```python
from build123d import *

# Parameters (mm, degrees)
SKETCH1_W           = 125
SKETCH1_H           = 6
BOSS_EXTRUDE1_DEPTH = 4
SKETCH2_R           = 1.15
CUT_EXTRUDE1_DEPTH  = 4
SKETCH4_W           = 6
SKETCH4_H           = 6
BOSS_EXTRUDE2_DEPTH = 10
SKETCH5_R           = 1.25
CUT_EXTRUDE2_DEPTH  = 10
SKETCH6_W           = 125
SKETCH6_H           = 6
CUT_EXTRUDE3_DEPTH  = 2
SKETCH7_R           = 1.5
CUT_EXTRUDE5_DEPTH  = 2
SKETCH8_R           = 1.5
CUT_EXTRUDE6_DEPTH  = 10
SKETCH9_R           = 1.5
CUT_EXTRUDE7_DEPTH  = 10
SKETCH10_W          = 6
SKETCH10_H          = 2
CUT_EXTRUDE8_DEPTH  = 20
SKETCH11_R          = 1.5
BOSS_EXTRUDE3_DEPTH = 2
SKETCH12_R          = 1.5
CUT_EXTRUDE9_DEPTH  = 2


with BuildPart() as part:
    # Sketch1 → Boss-Extrude1 (new body)
    with BuildSketch(Plane(origin=(0, 0, 0), x_dir=(1, 0, 0), z_dir=(0, 1, 0))):
        Rectangle(SKETCH1_W, SKETCH1_H)
    extrude(amount=BOSS_EXTRUDE1_DEPTH)

    # Sketch2 → Cut-Extrude1 (cut)
    with BuildSketch(Plane.XZ):
        with Locations(Location((0, 0, 0), (0, 0, 270))):
            Circle(SKETCH2_R)
    extrude(amount=-CUT_EXTRUDE1_DEPTH, mode=Mode.SUBTRACT)

    # Sketch4 → Boss-Extrude2 (add)
    with BuildSketch(Plane(origin=(62.5, 0, 0), x_dir=(0, 0, -1), z_dir=(1, 0, 0))):
        with Locations((0, 3)):
            Rectangle(SKETCH4_W, SKETCH4_H)
    extrude(amount=BOSS_EXTRUDE2_DEPTH)

    # Sketch5 → Cut-Extrude2 (cut)
    with BuildSketch(Plane(origin=(72.5, 0, 0), x_dir=(0, 0, -1), z_dir=(1, 0, 0))):
        with Locations((0, 3)):
            Circle(SKETCH5_R)
    extrude(amount=-CUT_EXTRUDE2_DEPTH, mode=Mode.SUBTRACT)

    # Sketch6 → Cut-Extrude3 (cut)
    with BuildSketch(Plane(origin=(0, 4, 0), x_dir=(1, 0, 0), z_dir=(0, 1, 0))):
        Rectangle(SKETCH6_W, SKETCH6_H)
    extrude(amount=-CUT_EXTRUDE3_DEPTH, mode=Mode.SUBTRACT)

    # Sketch7 → Cut-Extrude5 (cut)
    with BuildSketch(Plane(origin=(0, 2, 0), x_dir=(1, 0, 0), z_dir=(0, 1, 0))):
        with Locations(Location((0, 0, 0), (0, 0, 270))):
            Circle(SKETCH7_R)
    extrude(amount=-CUT_EXTRUDE5_DEPTH, mode=Mode.SUBTRACT)

    # Sketch8 → Cut-Extrude6 (cut)
    with BuildSketch(Plane(origin=(72.5, 0, 0), x_dir=(0, 0, -1), z_dir=(1, 0, 0))):
        with Locations((0, 3)):
            Circle(SKETCH8_R)
    extrude(amount=-CUT_EXTRUDE6_DEPTH, mode=Mode.SUBTRACT)

    # Sketch9 → Cut-Extrude7 (cut)
    with BuildSketch(Plane(origin=(0, 2, 0), x_dir=(1, 0, 0), z_dir=(0, 1, 0))):
        with Locations(Location((-57.5, 0, 0), (0, 0, 270))):
            Circle(SKETCH9_R)
    extrude(amount=-CUT_EXTRUDE7_DEPTH, mode=Mode.SUBTRACT)

    # Sketch10 → Cut-Extrude8 (cut)
    with BuildSketch(Plane.ZY.offset(62.5)):
        with Locations((0, 1)):
            Rectangle(SKETCH10_W, SKETCH10_H)
    extrude(amount=-CUT_EXTRUDE8_DEPTH, mode=Mode.SUBTRACT)

    # Sketch11 → Boss-Extrude3 (add)
    with BuildSketch(Plane(origin=(0, 2, 0), x_dir=(1, 0, 0), z_dir=(0, 1, 0))):
        Circle(SKETCH11_R)
    extrude(amount=-BOSS_EXTRUDE3_DEPTH)

    # Sketch12 → Cut-Extrude9 (cut)
    with BuildSketch(Plane(origin=(0, 2, 0), x_dir=(1, 0, 0), z_dir=(0, 1, 0))):
        with Locations(Location((7.5, 0, 0), (0, 0, 270))):
            Circle(SKETCH12_R)
    extrude(amount=-CUT_EXTRUDE9_DEPTH, mode=Mode.SUBTRACT)


solid = part.part
```
Model file for the job. Use its own axes, mm. A direction names the side the tool comes from. Coordinates: 2 decimals unless noted, no trailing zeros. Loops run counter-clockwise (first coordinate to the right, second up) from the corner with the lowest first, then second, coordinate; pieces in that order, holes last. Notation, with made-up numbers: (80, -8) - (103, -8) arc R27 ccw to (103, 31) - close; hole circle Ø2 at (77, 75). An arc over 180 degrees is marked (long way). Answer as a JSON object with one key per item and string values. Group by question number.
(1) Flat gauge pins, fed straight in: pin 1 (1.2 mm diameter, centred on y = 3, z = -1.5, fed in from -X); pin 2 (2.5 mm diameter, centred on y = 3, z = 0, fed in from +X); pin 3 (3.5 mm diameter, centred on x = 7.5, z = 0, fed in from +Y). Where does each tip first touch, or does it go through?
(2) Tool access for faces 4 (the face through (67.57, 1.536, 0.325)), 5 (the face through (27, 1.6, -3)), 6 (the face through (9.3, 2, 0)): list every direction of +Z, -Z, +X, -X, +Y, -Y with a clear straight run to the whole face (end or side of a thin tool).
(3) Two-plate mould, pull along X, no slides. Class faces 1 (the face through (6, 1, 0)), 2 (the face through (72.5, 4.4, 1.4)), 3 (the face through (14, 0, 0)): released by +X, released by -X, zero draft, split by the parting line, or undercut.
(4) Cut at B-B (x = 7.5). Give the cut face in (y, z), then the cut area to 3 significant figures.
(5) Cut at C-C (y = 3). Give the cut face in (x, z), then the cut area to 3 significant figures.
(6) Cut at D-D (x = -17). Give the cut face in (y, z), then the cut area to 3 significant figures.
(7) Probe line 1 along X through (y, z) = (0.85, 0); line 2 along Y through (x, z) = (66.75, 0); line 3 along X through (y, z) = (1.55, 0). List the from-to ranges inside material, lowest first.
(8) Cut at A-A (z = 0). Give the cut face in (x, y), then the cut area to 3 significant figures.
Geometry says:
{
 "1": {"pin 1": "stops at x = 62.5", "pin 2": "stops at x = 62.5", "pin 3": "stops at y = 2"},
 "2": {"face 4": "+X", "face 5": "-Z, +X, -X, +Y, -Y", "face 6": "+Z, -Z, -X, +Y"},
 "3": {"face 1": "undercut", "face 2": "released by +X", "face 3": "zero draft"},
 "4": {"outline": "(0, -3) - (2, -3) - (2, -1.5) - (0, -1.5) - close; (0, 1.5) - (2, 1.5) - (2, 3) - (0, 3) - close", "area": "6.00 mm^2"},
 "5": {"outline": "(62.5, -3) - (72.5, -3) - (72.5, -1.5) - (62.5, -1.5) - close; (62.5, 1.5) - (72.5, 1.5) - (72.5, 3) - (62.5, 3) - close", "area": "30.0 mm^2"},
 "6": {"outline": "(0, -3) - (2, -3) - (2, 3) - (0, 3) - close", "area": "12.0 mm^2"},
 "7": {"line 1": "x = -42.5 to 6, 9 to 72.5", "line 2": "y = 0 to 1.5, 4.5 to 6", "line 3": "x = -42.5 to 6, 9 to 62.5"},
 "8": {"outline": "(-42.5, 0) - (6, 0) - (6, 2) - (-42.5, 2) - close; (9, 0) - (72.5, 0) - (72.5, 1.5) - (62.5, 1.5) - (62.5, 2) - (9, 2) - close; (62.5, 4.5) - (72.5, 4.5) - (72.5, 6) - (62.5, 6) - close", "area": "234 mm^2"}
}
